Source: CAD feature listing. Evaluate the final solid. Frame: model axes, mm. A direction names the side the tool comes from. Coordinates: 2 decimals unless noted, no trailing zeros. Order: outer loops, then holes, each group sorted by start corner. A loop starts at its lowest first (then second) coordinate and runs counter-clockwise, first axis right, second up. Notation, with made-up numbers: (45, -27.75) -> (88, -27.75) arc R17 ccw to (88, -21.75) -> close; hole circle Ø1 at (-16, -5.5). An arc over 180 degrees is marked (long way). Write each question's results on one line, items separated by ' | '. Start each with the question number.
from build123d import *

# Parameters (mm, degrees)
EXTRUDE_1_DEPTH     = 9
SKETCH_2_R          = 5
CUT_EXTRUDE_1_DEPTH = 4.5
SKETCH_3_R          = 2
EXTRUDE_2_DEPTH     = 4
SKETCH_4_R          = 1
CUT_EXTRUDE_2_DEPTH = 10
SKETCH_5_R          = 1.75
CUT_EXTRUDE_3_DEPTH = 7
SKETCH_6_W          = 12.787856614
SKETCH_6_H          = 6.453658168
CUT_EXTRUDE_4_DEPTH = 2


with BuildPart() as part:
    # 草图1 → 凸台-拉伸1 (new body)
    with BuildSketch(Plane(origin=(0, 0, 0), x_dir=(1, 0, 0), z_dir=(0, 1, 0))):
        with BuildLine():
            Line((7.763932023, -2), (-7.763932023, -2))
            ThreePointArc((-7.763932023, -2), (-13, 0), (-7.763932023, 2))
            Line((-7.763932023, 2), (7.763932023, 2))
            ThreePointArc((7.763932023, 2), (13, 0), (7.763932023, -2))
        make_face()
    extrude(amount=EXTRUDE_1_DEPTH)

    # 草图2 → 切除-拉伸1 (cut)
    with BuildSketch(Plane(origin=(0, 9, 0), x_dir=(1, 0, 0), z_dir=(0, 1, 0))):
        with Locations((-10, 0)):
            Circle(SKETCH_2_R)
        with Locations((10, 0)):
            Circle(SKETCH_2_R)
    extrude(amount=-CUT_EXTRUDE_1_DEPTH, mode=Mode.SUBTRACT)

    # 草图3 → 凸台-拉伸2 (add)
    with BuildSketch(Plane(origin=(0, 4.5, 0), x_dir=(1, 0, 0), z_dir=(0, 1, 0))):
        with Locations((-10, 0)):
            Circle(SKETCH_3_R)
        with Locations((10, 0)):
            Circle(SKETCH_3_R)
    extrude(amount=EXTRUDE_2_DEPTH)

    # 草图4 → 切除-拉伸2 (cut, through all)
    with BuildSketch(Plane(origin=(0, 9, 0), x_dir=(1, 0, 0), z_dir=(0, 1, 0))):
        Circle(SKETCH_4_R)
    extrude(amount=-CUT_EXTRUDE_2_DEPTH, mode=Mode.SUBTRACT)

    # 草图5 → 切除-拉伸3 (cut)
    with BuildSketch(Plane(origin=(0, 9, 0), x_dir=(1, 0, 0), z_dir=(0, 1, 0))):
        Circle(SKETCH_5_R)
    extrude(amount=-CUT_EXTRUDE_3_DEPTH, mode=Mode.SUBTRACT)

    # 草图6 → 切除-拉伸4 (cut)
    with BuildSketch(Plane(origin=(0, 9, 0), x_dir=(1, 0, 0), z_dir=(0, 1, 0))):
        Rectangle(SKETCH_6_W, SKETCH_6_H)
    extrude(amount=-CUT_EXTRUDE_4_DEPTH, mode=Mode.SUBTRACT)


solid = part.part
(1) Section C-C on y = 1.25. Return the cut outline in (x, z).
(2) Section D-D on x = -10. Return the cut outline in (y, z).
(3) Draft query along X for faces 5 (the flat face through (-10, 8.5, 0)), 6 (the cylindrical face through (8.4, 6.5, 1.2)). Return one class per face: released by +X, released by -X, zero draft, split by the parting line, or undercut.
(4) Section A-A on y = 4.75. Return the cut outline in (x, z), then the cut area to 3 significant figures.
(5) Line query: L1, parallel to Z at x = 0, y = 0.55; L2, parallel to X at y = 3.7, z = 0; L3, parallel to Z at x = 0, y = 3.7. Output: solid intervals per line, ascending.
(6) First-contact query: P1, Ø5, axis at x = -1.5, y = 2.5, coming from the -Z side; P2, Ø3, axis at x = 0, z = 0, coming from the +Y side; P3, Ø3.5, axis at x = 1, y = 2.5, coming from the +Z side. Flat tips, straight axial feed; report the tip coordinate or a pass-through.
(7) Section B-B on z = 0. Return the cut outline in (x, y).
(8) Reachability of faces 1 (the flat face through (-1.3, 7, -1.4)), 2 (the flat face through (0, 3, 2)), 3 (the cylindrical face through (-11.6, 6.5, 1.2)), 4 (the flat face through (0, 3, -2)) from +Z, -Z, +X, -X, +Y, -Y: full face, straight path, thin tool, end or side. Return the list, or none.
Results list:
1) outline: (-7.76, -2) -> (7.76, -2) arc R3 ccw (long way) to (7.76, 2) -> (-7.76, 2) arc R3 ccw (long way) to start; hole circle Ø2 at (0, 0)
2) outline: (0, -3) -> (4.5, -3) -> (4.5, -2) -> (8.5, -2) -> (8.5, 2) -> (4.5, 2) -> (4.5, 3) -> (0, 3) -> close
3) face 5: zero draft | face 6: undercut
4) outline: circle Ø4 at (-10, 0); (-5.42, -2) -> (5.42, -2) arc R5 cw to (5.42, 2) -> (-5.42, 2) arc R5 cw to start; circle Ø4 at (10, 0); hole circle Ø3.5 at (0, 0) | area: 56.6 mm²
5) L1: z = -2 to -1, 1 to 2 | L2: x = -13 to -1.75, 1.75 to 13 | L3: z = -2 to -1.75, 1.75 to 2
6) P1: stops at z = -2 | P2: stops at y = 2 | P3: stops at z = 2
7) outline: (-13, 0) -> (-1, 0) -> (-1, 2) -> (-1.75, 2) -> (-1.75, 7) -> (-5, 7) -> (-5, 4.5) -> (-8, 4.5) -> (-8, 8.5) -> (-12, 8.5) -> (-12, 4.5) -> (-13, 4.5) -> close; (1, 0) -> (13, 0) -> (13, 4.5) -> (12, 4.5) -> (12, 8.5) -> (8, 8.5) -> (8, 4.5) -> (5, 4.5) -> (5, 7) -> (1.75, 7) -> (1.75, 2) -> (1, 2) -> close
8) face 1: +Z, -Z, +Y | face 2: +Z, +Y, -Y | face 3: +Y | face 4: -Z, +Y, -Y
